from build123d import *

# Parameters (mm, degrees)
SKETCH_1_W               = 50
SKETCH_1_H               = 40
EXTRUDE_1_DEPTH          = 40
CUT_EXTRUDE_1_DEPTH      = 30
CUT_EXTRUDE_2_DEPTH      = 20
CUT_EXTRUDE_3_DEPTH      = 10
CUT_EXTRUDE_4_DEPTH      = 1
CUT_EXTRUDE_4_DEPTH_BACK = 10


with BuildPart() as part:
    # 草圖1 → 填料-伸長1 (new body)
    with BuildSketch(Plane(origin=(0, 0, 0), x_dir=(1, 0, 0), z_dir=(0, 1, 0))):
        Rectangle(SKETCH_1_W, SKETCH_1_H)
    extrude(amount=EXTRUDE_1_DEPTH)

    # 草圖2 → 除料-伸長1 (cut)
    with BuildSketch(Plane(origin=(0, 40, 0), x_dir=(1, 0, 0), z_dir=(0, 1, 0))):
        Polygon((25, 0), (15, -20), (25, -20), align=None)
    extrude(amount=-CUT_EXTRUDE_1_DEPTH, mode=Mode.SUBTRACT)

    # 草圖3 → 除料-伸長2 (cut)
    with BuildSketch(Plane(origin=(0, 40, 0), x_dir=(1, 0, 0), z_dir=(0, 1, 0))):
        Polygon((25, 0), (15, 0), (5, -20), (15, -20), align=None)
    extrude(amount=-CUT_EXTRUDE_2_DEPTH, mode=Mode.SUBTRACT)

    # 草圖3<3> → 除料-伸長3 (cut)
    with BuildSketch(Plane(origin=(0, 40, 0), x_dir=(1, 0, 0), z_dir=(0, 1, 0))):
        Polygon((25, 0), (25, 20), (15, 0), align=None)
    extrude(amount=-CUT_EXTRUDE_3_DEPTH, mode=Mode.SUBTRACT)

    # 草圖4 → 除料-伸長4 (cut, two sides)
    with BuildSketch(Plane(origin=(0, 40, 0), x_dir=(1, 0, 0), z_dir=(0, 1, 0))) as cut_extrude_4_sk:
        Polygon((125, 0), (15, 0), (5, 0), (-5, -20), (5, -20), (115, -20), (311.77398202, -118.38699101), (321.77398202, -98.38699101), align=None)
    extrude(amount=CUT_EXTRUDE_4_DEPTH, mode=Mode.SUBTRACT)
    extrude(cut_extrude_4_sk.sketch, amount=-CUT_EXTRUDE_4_DEPTH_BACK, mode=Mode.SUBTRACT)


solid = part.part
The model under review builds one solid part; all positions refer to its coordinate system, in mm. A direction names the side the tool comes from. Round coordinates to 2 decimals unless told otherwise and drop trailing zeros. Order: outer loops, then holes, each group sorted by start corner. A loop starts at its lowest first (then second) coordinate and runs counter-clockwise, first axis right, second up. Notation, with made-up numbers: (7, 18.25) - (28, 18.25) arc R25 cw to (28, 51.25) - close; hole circle Ø5 at (80, 58.5). An arc over 180 degrees is marked (long way). Use one line per item in the form item = value.
Q1. Add section A-A on z = 7. Give the boundary of the cut face in (x, y), then the cut area to 4 significant figures.
Response values:
outline = (-25, 0) - (25, 0) - (25, 10) - (21.5, 10) - (21.5, 20) - (11.5, 20) - (11.5, 30) - (1.5, 30) - (1.5, 40) - (-25, 40) - close
area = 1,595 mm^2
Q2. To check wall thickness, follow line 1 (Z direction, x = 0, y = 32); line 2 (Z direction, x = 17, y = 27); line 3 (Y direction, x = 0.5, z = 18). State the ranges of each line that lie inside material, in increasing order.
Response values:
line_1 = -20 to 10
line_2 = -20 to 0
line_3 = 0 to 30
Q3. Add section C-C on y = 13.5. Give the boundary of the cut face in (x, z).
Response values:
outline = (-25, -20) - (25, -20) - (25, 0) - (15, 20) - (-25, 20) - close
Q4. Clearance check with flat-ended pins moving along their axes: P1, Ø4, axis at y = 13.5, z = 7, coming from the +X side; P2, Ø8, axis at x = 11, y = 37, coming from the +Z side; P3, Ø6, axis at x = 18, z = 12.5, coming from the +Y side. State where each tip first meets the part, or that it passes through.
Response values:
P1 = 22.5
P2 = 0
P3 = 20
Q5. Add section D-D on z = -12. Give the boundary of the cut face in (x, y).
Response values:
outline = (-25, 0) - (25, 0) - (25, 30) - (21, 30) - (21, 40) - (-25, 40) - close
Q6. Tool access review of faces 1 (the flat face through (-25, 20, 0)), 2 (the flat face through (20, 25, 0)): name each direction out of +Z, -Z, +X, -X, +Y, -Y from which nothing blocks a thin tool from reaching the whole face with its end or side.
Response values:
face_1 = +Z, -Z, -X, +Y, -Y
face_2 = +Z, +X, +Y
Q7. Add section B-B on x = 13.5. Give the boundary of the cut face in (y, z).
Response values:
outline = (0, -20) - (40, -20) - (40, 0) - (30, 0) - (30, 3) - (20, 3) - (20, 20) - (0, 20) - close
